The model under review builds one solid part; all positions refer to its coordinate system, in mm. A direction names the side the tool comes from. Give positions to 0.01 mm unless a question says otherwise; leave off trailing zeros. Loops run counter-clockwise (first coordinate to the right, second up) from the corner with the lowest first, then second, coordinate; pieces in that order, holes last. Notation, with made-up numbers: (23.25, 37) - (41.25, 37) arc R29 cw to (41.25, 68) - close; hole circle Ø9 at (16.25, 48). An arc over 180 degrees is marked (long way). Return JSON: item names as keys, results as strings. Group by question number.
```python
from build123d import *

# Parameters (mm, degrees)
F1_DEPTH = 9
F3_DEPTH = 12


with BuildPart() as f1:
    # F0 (on Front) → F1 (new body)
    with BuildSketch(Plane.XZ):
        with BuildLine():
            Line((0, 12), (0, 0))
            Line((0, 0), (3, 0))
            Line((3, 0), (3, 9.9171948475))
            Line((3, 9.9171948475), (3, 10))
            Line((3, 10), (3.0371407733, 10))
            ThreePointArc((3.0371407733, 10), (8.5, 13.5077309303), (13.9628592267, 10))
            Line((13.9628592267, 10), (14, 10))
            Line((14, 10), (14, 9.9171948475))
            Line((14, 9.9171948475), (14, 0))
            Line((14, 0), (17, 0))
            Line((17, 0), (17, 12))
            ThreePointArc((17, 12), (8.5, 15), (0, 12))
        make_face()
    extrude(amount=F1_DEPTH)

    # F2 (on Top) → F3 (join)
    with BuildSketch(Plane.XY):
        with BuildLine():
            ThreePointArc((0, -2), (-2.5, -4.5), (0, -7))
            Line((0, -7), (0, -5))
            ThreePointArc((0, -5), (-0.5, -4.5), (0, -4))
            Line((0, -4), (0, -2))
        make_face()
    extrude(amount=F3_DEPTH)


solid = f1.part
```
1) To check wall thickness, follow line 1 (X direction, y = -3, z = 5.5); line 2 (X direction, y = -1, z = 4.75); line 3 (Z direction, x = 11, y = -4.75). State the ranges of each line that lie inside material, in increasing order.
2) We need section C-C, the plane z = 13. Write out the cut boundary in (x, y), plus the area to 3 significant figures.
3) Draft analysis for pull direction X (two halves, no side actions). For faces 1 (the face through (-2.5, -4.4, 5.9)), 2 (the face through (0, -4.5, 6.1)), 3 (the face through (-1, -4, 12)), state which applies: +X half, -X half, draft (parallel to the pull), parting line (faces both ways), or undercut.
4) Tool access review of faces 4 (the face through (14, -4, 5)), 5 (the face through (0, -1, 6)), 6 (the face through (8.6, -4.4, 15)), 7 (the face through (1, -4, 0)), 8 (the face through (0, -8, 6)): name each direction out of +Z, -Z, +X, -X, +Y, -Y from which nothing blocks a thin tool from reaching the whole face with its end or side.
5) We need section B-B, the plane z = 10.5. Write out the cut boundary in (x, y), plus the area to 3 significant figures.
6) For pin 1 Ø1.2 at (x, y) = (-1.5, -5.5) entering from +Z; pin 2 Ø2 at (x, y) = (7.5, -7.5) entering from +Z; pin 3 Ø1.6 at (y, z) = (-8, 7) entering from -X; pin 4 Ø4 at (x, y) = (10.5, -6.5) entering from -Z, all flat-tipped, find the tip position at first contact; note any pin that passes through.
Findings:
{
 "1": {"line 1": "x = -2 to 3, 14 to 17", "line 2": "x = 0 to 3, 14 to 17", "line 3": "z = 12.96 to 14.77"},
 "2": {"outline": "(1.42, -9) - (6.08, -9) - (6.08, 0) - (1.42, 0) - close; (10.92, -9) - (15.58, -9) - (15.58, 0) - (10.92, 0) - close", "area": "84.0 mm^2"},
 "3": {"face 1": "-X half", "face 2": "undercut", "face 3": "draft"},
 "4": {"face 4": "-Z, +Y, -Y", "face 5": "+Z, -Z, -X, +Y", "face 6": "+Z, +Y, -Y", "face 7": "-Z, +X, -X, +Y, -Y", "face 8": "+Z, -Z, -X, -Y"},
 "5": {"outline": "(0, -9) - (3.29, -9) - (3.29, 0) - (0, 0) - (0, -2) arc R2.5 ccw to (0, -7) - close; (13.71, -9) - (17, -9) - (17, 0) - (13.71, 0) - close; hole (0, -5) - (0, -4) arc R0.5 ccw to start", "area": "68.7 mm^2"},
 "6": {"pin 1": "stops at z = 12", "pin 2": "stops at z = 15", "pin 3": "stops at x = 0", "pin 4": "stops at z = 11.98"}
}
